```python
from build123d import *

# Parameters (mm, degrees)
SKETCH1_R           = 10.5
BOSS_EXTRUDE1_DEPTH = 14
SKETCH2_R           = 7
BOSS_EXTRUDE2_DEPTH = 8
SKETCH3_R           = 2.5
CUT_EXTRUDE1_DEPTH  = 27.54241888
CUT_EXTRUDE2_START  = 1.5
SKETCH4_OUTSIDE_W   = 30.392
SKETCH4_OUTSIDE_H   = 30.392
SKETCH4_OUTSIDE_R   = 9.6623253
CUT_EXTRUDE2_DEPTH  = 11


with BuildPart() as part:
    # Sketch1 → Boss-Extrude1 (new body)
    with BuildSketch(Plane(origin=(0, 0, 0), x_dir=(1, 0, 0), z_dir=(0, 1, 0))):
        with Locations(Location((0, 0, 0), (0, 0, 270))):
            Circle(SKETCH1_R)
    extrude(amount=BOSS_EXTRUDE1_DEPTH)

    # Sketch2 → Boss-Extrude2 (add)
    with BuildSketch(Plane(origin=(0, 14, 0), x_dir=(1, 0, 0), z_dir=(0, 1, 0))):
        with Locations(Location((0, 0, 0), (0, 0, 270))):
            Circle(SKETCH2_R)
    extrude(amount=BOSS_EXTRUDE2_DEPTH)

    # Sketch3 → Cut-Extrude1 (cut, through all)
    with BuildSketch(Plane(origin=(0, 22, 0), x_dir=(1, 0, 0), z_dir=(0, 1, 0))):
        with Locations(Location((0, 0, 0), (0, 0, 270))):
            Circle(SKETCH3_R)
    extrude(amount=-CUT_EXTRUDE1_DEPTH, mode=Mode.SUBTRACT)

    # Sketch4 outside → Cut-Extrude2 (cut)
    with BuildSketch(Plane(origin=(0, 0, 0), x_dir=(1, 0, 0), z_dir=(0, 1, 0)).offset(CUT_EXTRUDE2_START)):
        Rectangle(SKETCH4_OUTSIDE_W, SKETCH4_OUTSIDE_H)
        with Locations(Location((0, 0, 0), (0, 0, 270))):
            Circle(SKETCH4_OUTSIDE_R, mode=Mode.SUBTRACT)
    extrude(amount=CUT_EXTRUDE2_DEPTH, mode=Mode.SUBTRACT)


solid = part.part
```
Here's how the part is built. I have some questions about the finished solid (model axes, mm). A direction names the side the tool comes from. Give positions to 0.01 mm unless a question says otherwise; leave off trailing zeros. Order: outer loops, then holes, each group sorted by start corner. A loop starts at its lowest first (then second) coordinate and runs counter-clockwise, first axis right, second up. Notation, with made-up numbers: (-21.75, -3.75) -> (24.25, -3.75) arc R21 cw to (24.25, 22.25) -> close; hole circle Ø1 at (-30.5, 55.5). An arc over 180 degrees is marked (long way). Use CSV: the item, a comma, the result in double quotes. Start each with the question number.
Item 1: If I drill on probe 1 along X at (y, z) = (16.5, 0); probe 2 along X at (y, z) = (5.5, 0); probe 3 along Z at (x, y) = (2.25, 4.75), over which ranges is the centre line in solid material (lowest first)? Write a range as [from, to].
Item 2: Suppose I cut it at D-D (x = 5.5). List the corners of the cut face in (y, z) for me, and give its area (3 significant figures).
Item 3: Suppose I cut it at B-B (z = 0). List the corners of the cut face in (x, y) for me, and give its area (3 significant figures).
Item 4: Suppose I cut it at C-C (y = 15.5). List the corners of the cut face in (x, z) for me.
Item 5: Thinking about a two-plate mould opening in Z: for faces 4 (the flat face through (0, 22, 3)), 5 (the cylindrical face through (3.2, 13.2, 10)), 6 (the cylindrical face through (-2.44, 11.15, -0.54)), which applies, pulls with the +Z half, pulls with the -Z half, needs draft (parallel to the pull), parting line crosses it, or undercut?
Item 6: I'm going to push flat-ended pins straight in: P1, Ø1.5, axis at x = -2, y = 14, coming from the +Z side; P2, Ø10, axis at y = 6.5, z = 8.5, coming from the -X side; P3, Ø2, axis at y = 9, z = -2, coming from the -X side. Where does each tip first touch, or does it pass through?
Item 7: Suppose I cut it at A-A (x = 0). List the corners of the cut face in (y, z) for me.
Item 8: On a 3-axis mill with a long thin cutter (end or side, diameter ignored), from which of +Z, -Z, +X, -X, +Y, -Y can I reach the whole of each face in a straight line? I mean faces 1 (the flat face through (5, 12.5, 9)), 2 (the cylindrical face through (-6.834, 17.944, -1.517)), 3 (the flat face through (-2, 0, 2)). Say none if no direction works.
Answer block:
1,probe 1,"x = [-7, -2.5], [2.5, 7]"
1,probe 2,"x = [-9.66, -2.5], [2.5, 9.66]"
1,probe 3,"z = [-9.4, -1.09], [1.09, 9.4]"
2,outline,"(0, -8.94) -> (1.5, -8.94) -> (1.5, -7.94) -> (12.5, -7.94) -> (12.5, -8.94) -> (14, -8.94) -> (14, -4.33) -> (22, -4.33) -> (22, 4.33) -> (14, 4.33) -> (14, 8.94) -> (12.5, 8.94) -> (12.5, 7.94) -> (1.5, 7.94) -> (1.5, 8.94) -> (0, 8.94) -> close"
2,area,"298 mm^2"
3,outline,"(-10.5, 0) -> (-2.5, 0) -> (-2.5, 22) -> (-7, 22) -> (-7, 14) -> (-10.5, 14) -> (-10.5, 12.5) -> (-9.66, 12.5) -> (-9.66, 1.5) -> (-10.5, 1.5) -> close; (2.5, 0) -> (10.5, 0) -> (10.5, 1.5) -> (9.66, 1.5) -> (9.66, 12.5) -> (10.5, 12.5) -> (10.5, 14) -> (7, 14) -> (7, 22) -> (2.5, 22) -> close"
3,area,"278 mm^2"
4,outline,"circle Ø14 at (0, 0); hole circle Ø5 at (0, 0)"
5,face 4,"needs draft"
5,face 5,"parting line crosses it"
5,face 6,"undercut"
6,P1,"stops at z = 10.43"
6,P2,"stops at x = -9.01"
6,P3,"stops at x = -9.61"
7,outline,"(0, -10.5) -> (1.5, -10.5) -> (1.5, -9.66) -> (12.5, -9.66) -> (12.5, -10.5) -> (14, -10.5) -> (14, -7) -> (22, -7) -> (22, -2.5) -> (0, -2.5) -> close; (0, 2.5) -> (22, 2.5) -> (22, 7) -> (14, 7) -> (14, 10.5) -> (12.5, 10.5) -> (12.5, 9.66) -> (1.5, 9.66) -> (1.5, 10.5) -> (0, 10.5) -> close"
8,face 1,"none"
8,face 2,"+Y"
8,face 3,"+Z, -Z, +X, -X, -Y"
